Check sheet for the modelled part. Datum: model origin and axes. Units: mm. Coordinates: 2 decimals unless noted, no trailing zeros. Loops run counter-clockwise (first coordinate to the right, second up) from the corner with the lowest first, then second, coordinate; pieces in that order, holes last. Notation, with made-up numbers: M -12.5,31.5 L 37.5,31.5 A18 ccw 37.5,40.5 Z; hole C 39,64 d1. An arc over 180 degrees is marked long. Return JSON: item names as keys, results as strings.
Autodesk Inventor part; units mm, degrees
ref_plane "Work Plane1" through (-69.3675, -78.2107, 0) normal (-1, 0, 0) x (0, 0, 1)
ref_plane "YZ Plane" through (0, 0, 0) normal (1, 0, 0) x (0, 1, 0)
ref_plane "XZ Plane" through (0, 0, 0) normal (0, 1, 0) x (-1, 0, 0)
sketch "Sketch1" plane through (0, 0, 0) normal (1, 0, 0) x (0, 1, 0)
  circle A0 centre (0, 0) radius 3
  circle A1 centre (0, 0) radius 7.5
  dimension "d0" = 6
  dimension "d1" = 15
extrude "Extrusion1" add sketch "Sketch1" along normal blind 14
sketch "Sketch2" plane through (0, 0, 0) normal (0, 0, 1) x (1, 0, 0)
  line L0 (14, -7.5) -> (14, 7.5)
  line L1 (0, -7.5) -> (0, 7.5)
  line L2 (0, -7.5) -> (14, -7.5)
  line L3 (7, -7.5) -> (-63.7107, -78.2107)
  line L4 (13.2599, -6.897) -> (-46.7401, -66.897)
  line L5 (3.7119, -5.1312) -> (-52.397, -61.2401)
  line L6 (-52.397, -61.2401) -> (-58.0538, -66.897)
  line L7 (-63.7107, -78.2107) -> (-58.0538, -78.2107)
  line L8 (-63.7107, -78.2107) -> (-69.3675, -78.2107)
  line L9 (-58.0538, -78.2107) -> (-46.7401, -66.897)
  line L10 (-58.0538, -66.897) -> (-69.3675, -78.2107)
  line L11 (3.7119, -5.1312) -> (12.583, -5.1312)
  line L12 (13.2599, -6.897) -> (12.583, -5.1312)
  point P0 (0, 0)
  point P1 (-58.0538, -78.2107)
  point P2 (1.3431, -7.5)
  point P3 (12.6569, -7.5)
  dimension "d4" = 100
  dimension "d5" = 45
  dimension "d6" = 4
  dimension "d7" = 4
  dimension "d10" = 8.871
  dimension "d12" = 60
extrude "Extrusion2" add sketch "Sketch2" along normal mid plane 8
extrude "Extrusion3" add sketch "Sketch1" along normal blind 2 contours A0
ref_plane "Work Plane1" through (-69.3675, -78.2107, 0) normal (-1, 0, 0) x (0, 0, 1)
sketch "Sketch3" plane through (-69.3675, -78.2107, 0) normal (-1, 0, 0) x (0, 0, 1)
  arc A0 (-4, 71.8664) -> (4, 71.8664) centre (0, 78.2107) ccw
  line L0 (-4, 0) -> (-4, 71.8664)
  line L1 (-4, 0) -> (4, 0)
  line L2 (4, 71.8664) -> (4, 0)
  circle A1 centre (0, -5.241) radius 7.5
  circle A2 centre (0, -5.241) radius 3
  line L3 (0, -32.4313) -> (0, 105.401)
  point P0 (0, 0)
  dimension "d15" = 15
  dimension "d16" = 6
  dimension "d17" = 5.241
extrude "Extrusion4" add sketch "Sketch3" against normal blind 9 contours A1 L3 L1 L0 | L0 L1 L3 A2 A1 | A1 L2 L1 L3 | L3 A2 L1 L2 A1
sketch "Sketch4" plane through (-60.3675, -78.2107, 0) normal (1, 0, 0) x (0, 0, -1)
  circle A0 centre (0, -5.241) radius 3
  circle A1 centre (0, -5.241) radius 5
  point P0 (0, 78.2107)
  dimension "d20" = 10
extrude "Extrusion5" cut sketch "Sketch4" along normal blind 9 and the other way blind 4
properties part number "Conector"
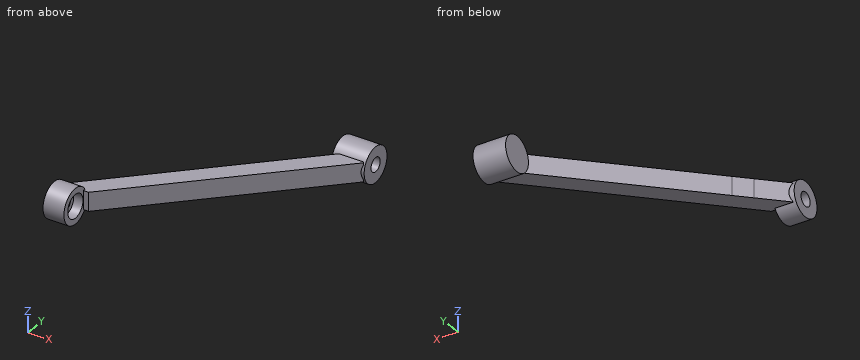
1) Section check B-B on y = 0. Record the cut outline in (x, z).
Answers:
{"outline": "M 0,-7.5 L 14,-7.5 L 14,-3 L 2,-3 L 2,3 L 14,3 L 14,7.5 L 0,7.5 Z"}
2) Section check D-D on x = -31.5. Record the cut outline in (y, z), then the cut area to 3 significant figures.
Answers:
{"outline": "M -51.66,-4 L -40.34,-4 L -40.34,4 L -51.66,4 Z", "area": "90.5 mm²"}
3) Scan lines: line 1 along Y through (x, z) = (-67.6, 0); line 2 along Z through (x, y) = (9.75, 0); line 3 along Z through (x, y) = (0, -18.5). Record each from-to range of solid material in increasing order. Write a range as [from, to].
Answers:
{"line 1": "[-90.95, -86.45], [-80.45, -75.95]", "line 2": "[-7.5, -3], [3, 7.5]", "line 3": "[-4, 4]"}
4) Section check C-C on x = -62.5. Record the cut outline in (y, z), then the cut area to 3 significant figures.
Answers:
{"outline": "M -77.11,-4 L -71.34,-4 L -71.34,4 L -77.11,4 A7.5 ccw long Z; hole C -83.45,0 d10", "area": "138 mm²"}
5) Go/stop test with flat-tipped pins: pin 1 Ø1 at (x, z) = (0.5, 0.5) entering from +Y; pin 2 Ø3 at (x, z) = (-54.5, 2.5) entering from -Y; pin 3 Ø4 at (y, z) = (-34.5, 2) entering from +X; pin 4 Ø4 at (y, z) = (-35.5, 1) entering from +X. Record where each tip stops, or that it passes through.
Answers:
{"pin 1": "y = 7.5", "pin 2": "y = -76.16", "pin 3": "x = -12.34", "pin 4": "x = -13.34"}
6) Section check A-A on z = 0. Record the cut outline in (x, y), then the cut area to 3 significant figures.
Answers:
{"outline": "M -69.37,-90.95 L -60.37,-90.95 L -60.37,-88.45 L -64.37,-88.45 L -64.37,-86.45 L -69.37,-86.45 Z; M -69.37,-80.45 L -64.37,-80.45 L -64.37,-78.45 L -60.37,-78.45 L -60.37,-78.21 L -58.05,-78.21 L 12.66,-7.5 L 14,-7.5 L 14,-3 L 2,-3 L 2,3 L 14,3 L 14,7.5 L 0,7.5 L 0,-7.5 L 1.34,-7.5 L -52.4,-61.24 L -58.05,-66.9 L -67.11,-75.95 L -69.37,-75.95 Z", "area": "985 mm²"}
